Input: part model. Units: mm. Frame: model coordinates. A direction names the side the tool comes from. Coordinates: 2 decimals unless noted, no trailing zeros. Order: outer loops, then holes, each group sorted by start corner. A loop starts at its lowest first (then second) coordinate and runs counter-clockwise, first axis right, second up. Notation, with made-up numbers: (78, -29) -> (110, -29) arc R15 cw to (110, -23) -> close; hole circle Ø7 at (45, 1.25). An arc over 180 degrees is marked (long way). One line per question, with ' | ' between items.
```python
from build123d import *

# Parameters (mm, degrees)
SKETCH_1_R      = 1.65
EXTRUDE_1_DEPTH = 3
SKETCH_2_R      = 5
SKETCH_2_R_2    = 1.65
EXTRUDE_2_DEPTH = 8.5


with BuildPart() as part:
    # 草圖1 → 填料-伸長1 (new body)
    with BuildSketch(Plane.XY):
        with BuildLine():
            Line((0, 5), (51, 5))
            ThreePointArc((51, 5), (56, 0), (51, -5))
            Line((51, -5), (0, -5))
            ThreePointArc((0, -5), (-5, 0), (0, 5))
        make_face()
        Circle(SKETCH_1_R, mode=Mode.SUBTRACT)
        with Locations((51, 0)):
            Circle(SKETCH_1_R, mode=Mode.SUBTRACT)
    extrude(amount=EXTRUDE_1_DEPTH)

    # 草圖2 → 填料-伸長2 (add)
    with BuildSketch(Plane(origin=(0, 0, 0), x_dir=(-1, 0, 0), z_dir=(0, 0, -1))):
        with Locations((-51, 0)):
            Circle(SKETCH_2_R)
        with Locations((-51, 0)):
            Circle(SKETCH_2_R_2, mode=Mode.SUBTRACT)
    extrude(amount=EXTRUDE_2_DEPTH)


solid = part.part
```
1. Mould query, pull axis Y, two halves, no side actions, for faces 3 (the face through (-1.216, 1.115, 1.479)), 4 (the face through (26, -5, 1)), 5 (the face through (-5, 0, 1)), 6 (the face through (49, 0, -8.5)). Classes: released by +Y, released by -Y, zero draft, split by the parting line, or undercut.
Recorded:
face 3: undercut | face 4: released by -Y | face 5: split by the parting line | face 6: zero draft
2. Access query for faces 1 (the face through (56, 0, -3)), 2 (the face through (26, 0, 3)). Directions: +Z, -Z, +X, -X, +Y, -Y. A direction counts if a zero-diameter tool reaches every point of the face in a straight line with its end or side. Return the directions, or none.
Recorded:
face 1: -Z | face 2: +Z, +X, -X, +Y, -Y
3. Cut plane C-C, the plane z = 2.25. Return loops of the section in (x, y), and give its area (3 significant figures).
Recorded:
outline: (0, -5) -> (51, -5) arc R5 ccw to (51, 5) -> (0, 5) arc R5 ccw to start; hole circle Ø3.3 at (0, 0); hole circle Ø3.3 at (51, 0) | area: 571 mm^2
4. Cut plane D-D, the plane z = -3. Return loops of the section in (x, y), and give its area (3 significant figures).
Recorded:
outline: circle Ø10 at (51, 0); hole circle Ø3.3 at (51, 0) | area: 70.0 mm^2
5. Cut plane A-A, the plane y = 0. Return loops of the section in (x, z).
Recorded:
outline: (-5, 0) -> (-1.65, 0) -> (-1.65, 3) -> (-5, 3) -> close; (1.65, 0) -> (46, 0) -> (46, -8.5) -> (49.35, -8.5) -> (49.35, 3) -> (1.65, 3) -> close; (52.65, -8.5) -> (56, -8.5) -> (56, 3) -> (52.65, 3) -> close
6. Cut plane B-B, the plane x = 48. Return loops of the section in (y, z), and give its area (3 significant figures).
Recorded:
outline: (-5, 0) -> (-4, 0) -> (-4, -8.5) -> (4, -8.5) -> (4, 0) -> (5, 0) -> (5, 3) -> (-5, 3) -> close | area: 98.0 mm^2
7. Pin query (flat end, axial travel): pin 1 Ø4 at (y, z) = (3.5, -4) entering from -X; pin 2 Ø4 at (x, y) = (34.5, 0) entering from -Z. Return the tip coordinate at first contact, or that it passes through.
Recorded:
pin 1: stops at x = 46.23 | pin 2: stops at z = 0
8. Ray query, line 1 (Y direction, x = 51, z = -5.5); line 2 (X direction, y = 0, z = -4.75); line 3 (Z direction, x = 43, y = 1.5). Return the intervals inside material, ascending. Write a range as [from, to].
Recorded:
line 1: y = [-5, -1.65], [1.65, 5] | line 2: x = [46, 49.35], [52.65, 56] | line 3: z = [0, 3]
